The listing builds one solid part. Answer for the finished solid, in the listing's coordinates (mm). A direction names the side the tool comes from. Give positions to 0.01 mm unless a question says otherwise; leave off trailing zeros. Write each loop counter-clockwise with the first axis right and the second up, starting at its lowest first coordinate (ties: lowest second). Pieces come first, ordered by that corner, then holes. Notation, with made-up numbers: M 41.25,53.25 L 100.25,53.25 A18 ccw 100.25,68.25 Z; hole C -16,-19 d6. An arc over 180 degrees is marked long. Return JSON: item names as keys, results as strings.
from build123d import *

# Parameters (mm, degrees)
SKETCH_1_W          = 10
SKETCH_1_H          = 10
SKETCH_1_W_2        = 8
SKETCH_1_H_2        = 8
EXTRUDE_1_DEPTH     = 84
SKETCH_3_R          = 1.5
CUT_EXTRUDE_2_DEPTH = 10


with BuildPart() as part:
    # 草图1 → 拉伸-薄壁1 (new body)
    with BuildSketch(Plane.XY):
        with Locations((-72.076665045, -5)):
            Rectangle(SKETCH_1_W, SKETCH_1_H)
        with Locations((-72.076665045, -5)):
            Rectangle(SKETCH_1_W_2, SKETCH_1_H_2, mode=Mode.SUBTRACT)
    extrude(amount=EXTRUDE_1_DEPTH)

    # 草图3 → 切除-拉伸2 (cut)
    with BuildSketch(Plane.XZ.offset(10)):
        with Locations((-72.076665045, 5)):
            Circle(SKETCH_3_R)
        with Locations((-72.076665045, 79)):
            Circle(SKETCH_3_R)
        with Locations((-72.076665045, 69)):
            Circle(SKETCH_3_R)
        with Locations((-72.076665045, 15)):
            Circle(SKETCH_3_R)
    extrude(amount=-CUT_EXTRUDE_2_DEPTH, mode=Mode.SUBTRACT)


solid = part.part
Item 1: Determine the mould class of faces 1 (the flat face through (-67.7, -4.9, 84)), 2 (the cylindrical face through (-70.646, -9.507, 69.451)), 3 (the cylindrical face through (-70.646, -9.507, 5.451)), 4 (the flat face through (-67.077, -5, 41)) for opening direction Z: +Z half, -Z half, draft (parallel to the pull), parting line (faces both ways), or undercut.
Geometry results:
{"face 1": "+Z half", "face 2": "undercut", "face 3": "undercut", "face 4": "draft"}
Item 2: A cutting plane is placed at B-B, the plane z = 15. Write down the section's boundary in (x, y), plus the area to 3 significant figures.
Geometry results:
{"outline": "M -77.08,-10 L -73.58,-10 L -73.58,-9 L -76.08,-9 L -76.08,-1 L -73.58,-1 L -73.58,0 L -77.08,0 Z; M -70.58,-10 L -67.08,-10 L -67.08,0 L -70.58,0 L -70.58,-1 L -68.08,-1 L -68.08,-9 L -70.58,-9 Z", "area": "30.0 mm2"}
Item 3: A cutting plane is placed at A-A, the plane x = -69.25. Write down the section's boundary in (y, z), plus the area to 3 significant figures.
Geometry results:
{"outline": "M -10,0 L -9,0 L -9,84 L -10,84 Z; M -1,0 L 0,0 L 0,84 L -1,84 Z", "area": "168 mm2"}
Item 4: Find the intervals of material crossed by line 1 (X direction, y = -9.3, z = 69); line 2 (X direction, y = -7, z = 72); line 3 (Y direction, x = -72.5, z = 25.5), in increasing order.
Geometry results:
{"line 1": "x = -77.08 to -73.58, -70.58 to -67.08", "line 2": "x = -77.08 to -76.08, -68.08 to -67.08", "line 3": "y = -10 to -9, -1 to 0"}
Item 5: A cutting plane is placed at D-D, the plane z = 62. Write down the section's boundary in (x, y).
Geometry results:
{"outline": "M -77.08,-10 L -67.08,-10 L -67.08,0 L -77.08,0 Z; hole M -76.08,-9 L -68.08,-9 L -68.08,-1 L -76.08,-1 Z"}
Item 6: Given pin 1 Ø2 at (x, y) = (-70.5, -3) entering from +Z, flat-ended and moving along its own axis, determine where the tip first touches the part or whether it passes through.
Geometry results:
{"pin 1": "passes through"}
Item 7: A cutting plane is placed at C-C, the plane y = -6.25. Write down the section's boundary in (x, z), plus the area to 3 significant figures.
Geometry results:
{"outline": "M -77.08,0 L -76.08,0 L -76.08,84 L -77.08,84 Z; M -68.08,0 L -67.08,0 L -67.08,84 L -68.08,84 Z", "area": "168 mm2"}
Item 8: Which of the six approach directions +Z, -Z, +X, -X, +Y, -Y give full straight-line access (tool end or side, diameter ignored) to faces 5 (the cylindrical face through (-71.27, -0.507, 80.265)), 6 (the flat face through (-72, -9, 41))?
Geometry results:
{"face 5": "+Y, -Y", "face 6": "+Z, -Z"}
